from build123d import *

# Parameters (mm, degrees)
BOSS_EXTRUDE1_DEPTH = 4
SKETCH2_R           = 2.75
CUT_EXTRUDE1_DEPTH  = 3
SKETCH3_R           = 2.35
BOSS_EXTRUDE2_DEPTH = 4
CHAMFER1_SIZE       = 1
CUT_EXTRUDE2_DEPTH  = 2.5
SKETCH6_W           = 2.7
SKETCH6_H           = 2.7
BOSS_EXTRUDE3_DEPTH = 4
CHAMFER2_SIZE       = 0.74


with BuildPart() as part:
    # Sketch1 → Boss-Extrude1 (new body)
    with BuildSketch(Plane.XY):
        with BuildLine():
            Line((120.3, 160), (146.661746787, 160))
            ThreePointArc((146.661746787, 160), (148.349682778, 160.578969808), (149.32688133, 162.072093023))
            ThreePointArc((149.32688133, 162.072093023), (152.169640756, 166.415724194), (157.08, 168.1))
            Line((157.08, 168.1), (277.08, 168.1))
            ThreePointArc((277.08, 168.1), (281.990359244, 166.415724194), (284.83311867, 162.072093023))
            ThreePointArc((284.83311867, 162.072093023), (285.810317222, 160.578969808), (287.498253213, 160))
            Line((287.498253213, 160), (370, 160))
            ThreePointArc((370, 160), (377.071067812, 157.071067812), (380, 150))
            Line((380, 150), (380, 10))
            ThreePointArc((380, 10), (377.071067812, 2.928932188), (370, 0))
            Line((370, 0), (287.498253213, 0))
            ThreePointArc((287.498253213, 0), (285.810317222, -0.578969808), (284.83311867, -2.072093023))
            ThreePointArc((284.83311867, -2.072093023), (281.990359244, -6.415724194), (277.08, -8.1))
            Line((277.08, -8.1), (157.08, -8.1))
            ThreePointArc((157.08, -8.1), (152.169640756, -6.415724194), (149.32688133, -2.072093023))
            ThreePointArc((149.32688133, -2.072093023), (148.349682778, -0.578969808), (146.661746787, 0))
            Line((146.661746787, 0), (120.3, 0))
            Line((120.3, 0), (120.3, 160))
        make_face()
    extrude(amount=BOSS_EXTRUDE1_DEPTH)

    # Sketch2 → Cut-Extrude1 (cut)
    with BuildSketch(Plane(origin=(0, 0, 0), x_dir=(-1, 0, 0), z_dir=(0, 0, -1))):
        with Locations((-126.25, 8.75)):
            Circle(SKETCH2_R)
        with Locations((-126.25, 151.25)):
            Circle(SKETCH2_R)
        with Locations((-370, 10)):
            Circle(SKETCH2_R)
        with Locations((-370, 150)):
            Circle(SKETCH2_R)
    extrude(amount=-CUT_EXTRUDE1_DEPTH, mode=Mode.SUBTRACT)

    # Sketch3 → Boss-Extrude2 (add)
    with BuildSketch(Plane(origin=(0, 0, 0), x_dir=(-1, 0, 0), z_dir=(0, 0, -1))):
        with Locations((-157.08, -0.1)):
            Circle(SKETCH3_R)
        with Locations((-157.08, 160.1)):
            Circle(SKETCH3_R)
        with Locations((-277.08, 160.1)):
            Circle(SKETCH3_R)
        with Locations((-277.08, -0.1)):
            Circle(SKETCH3_R)
    extrude(amount=BOSS_EXTRUDE2_DEPTH)

    # Chamfer1
    chamfer1_edges = [part.edges().sort_by_distance(p)[0] for p in [
        (159.43, -0.1, -4),
        (159.43, 160.1, -4),
        (279.43, 160.1, -4),
        (279.43, -0.1, -4),
    ]]
    chamfer(chamfer1_edges, length=CHAMFER1_SIZE)

    # Sketch4 → Cut-Extrude2 (cut)
    with BuildSketch(Plane(origin=(0, 0, 0), x_dir=(-1, 0, 0), z_dir=(0, 0, -1))):
        with BuildLine():
            ThreePointArc((-370, 15.75), (-365.934136008, 14.065863992), (-364.25, 10))
            Line((-364.25, 10), (-364.25, 3))
            Line((-364.25, 3), (-272.08, 3))
            Line((-272.08, 3), (-272.08, -5.1))
            Line((-272.08, -5.1), (-162.08, -5.1))
            Line((-162.08, -5.1), (-162.08, 3))
            Line((-162.08, 3), (-132, 3))
            Line((-132, 3), (-132, 8.75))
            ThreePointArc((-132, 8.75), (-130.315863992, 12.815863992), (-126.25, 14.5))
            Line((-126.25, 14.5), (-122.867487478, 14.5))
            Line((-122.867487478, 14.5), (-122.867487478, 145.5))
            Line((-122.867487478, 145.5), (-126.25, 145.5))
            ThreePointArc((-126.25, 145.5), (-130.315863992, 147.184136008), (-132, 151.25))
            Line((-132, 151.25), (-132, 157))
            Line((-132, 157), (-162.08, 157))
            Line((-162.08, 157), (-162.08, 165.1))
            Line((-162.08, 165.1), (-272.08, 165.1))
            Line((-272.08, 165.1), (-272.08, 157))
            Line((-272.08, 157), (-364.25, 157))
            Line((-364.25, 157), (-364.25, 150))
            ThreePointArc((-364.25, 150), (-365.934136008, 145.934136008), (-370, 144.25))
            Line((-370, 144.25), (-374, 144.25))
            Line((-374, 144.25), (-374, 141.25))
            Line((-374, 141.25), (-377, 141.25))
            Line((-377, 141.25), (-377, 18.75))
            Line((-377, 18.75), (-374, 18.75))
            Line((-374, 18.75), (-374, 15.75))
            Line((-374, 15.75), (-370, 15.75))
        make_face()
    extrude(amount=-CUT_EXTRUDE2_DEPTH, mode=Mode.SUBTRACT)

    # Sketch6 → Boss-Extrude3 (add)
    with BuildSketch(Plane(origin=(0, 0, 0), x_dir=(-1, 0, 0), z_dir=(0, 0, -1))):
        with Locations((-375.35, 17.4)):
            Rectangle(SKETCH6_W, SKETCH6_H)
        with Locations((-375.35, 142.6)):
            Rectangle(SKETCH6_W, SKETCH6_H)
    extrude(amount=BOSS_EXTRUDE3_DEPTH)

    # Chamfer2
    chamfer2_edges = [part.edges().sort_by_distance(p)[0] for p in [
        (376.7, 16.05, -2),
        (376.7, 17.4, -4),
        (375.35, 16.05, -4),
        (376.7, 143.95, -2),
        (375.35, 143.95, -4),
        (376.7, 142.6, -4),
    ]]
    chamfer(chamfer2_edges, length=CHAMFER2_SIZE)


solid = part.part
Here's how the part is built. I have some questions about the finished solid (model axes, mm). A direction names the side the tool comes from. Coordinates: 2 decimals unless noted, no trailing zeros. Write each loop counter-clockwise with the first axis right and the second up, starting at its lowest first coordinate (ties: lowest second). Pieces come first, ordered by that corner, then holes.
Item 1: On a 3-axis mill with a long thin cutter (end or side, diameter ignored), from which of +Z, -Z, +X, -X, +Y, -Y can I reach the whole of each face in a straight line? I mean faces 5 (the cylindrical face through (130.27, 147.14, 1.23)), 6 (the cylindrical face through (282.05, -6.37, 1.97)). Say none if no direction works.
Item 2: I want a section at B-B on y = 52. Write out the boundary of the cut face in (x, z).
Item 3: If we mould it in two halves opening along Y, with no side actions, what happens to faces 1 (the cylindrical face through (130.36, 12.77, 1.23)), 2 (the flat face through (370, 10, 3)), 3 (the cylindrical face through (376.99, 157.15, 1.97)), 4 (the cylindrical face through (152.23, -6.46, 1.97))? For each: +Y half, -Y half, draft (parallel to the pull), parting line (faces both ways), or undercut.
Item 4: Will these pins go through, and if not, where does the flat tip stop? pin 1 (1.5 mm diameter, centred on y = 143, z = -0.5, fed in from -X); pin 2 (1.2 mm diameter, centred on x = 372, z = 1.5, fed in from -Y); pin 3 (4.5 mm diameter, centred on x = 135, z = 2, fed in from -Y); pin 4 (2 mm diameter, centred on y = 154, z = 1, fed in from +X).
Item 5: I want a section at A-A on x = 224. Write out the boundary of the cut face in (y, z).
Item 6: I want a section at C-C on z = 1.25. Count the separate pieces of the cut face and the enclosed holes in it, and give its area (3 significant figures).
Item 7: If I drill on line 1 (Y direction, x = 370, z = 0.8); line 2 (Y direction, x = 126.25, z = 0.8); line 3 (X direction, y = 128, z = 1), over which ranges is the centre line in solid material (lowest first)?
Findings below:
1. face 5: -Z
1. face 6: +Z, -Z, +X, -Y
2. outline: (120.3, 0) - (122.87, 0) - (122.87, 2.5) - (377, 2.5) - (377, 0) - (380, 0) - (380, 4) - (120.3, 4) - close
3. face 1: undercut
3. face 2: undercut
3. face 3: +Y half
3. face 4: -Y half
4. pin 1: stops at x = 120.3
4. pin 2: stops at y = 0.1
4. pin 3: stops at y = 0
4. pin 4: stops at x = 379.54
5. outline: (-8.1, 0) - (-5.1, 0) - (-5.1, 2.5) - (165.1, 2.5) - (165.1, 0) - (168.1, 0) - (168.1, 4) - (-8.1, 4) - close
6. separate pieces: 1
6. enclosed holes: 5
6. area: 3,170 mm2
7. line 1: y = 0 to 7.25, 12.75 to 15.75, 144.25 to 147.25, 152.75 to 160
7. line 2: y = 0 to 6, 11.5 to 14.5, 145.5 to 148.5, 154 to 160
7. line 3: x = 120.3 to 122.87, 377 to 380
